from build123d import *

# Parameters (mm, degrees)
F0_R     = 2.5
F0_R_2   = 5
F0_R_3   = 2
F0_W     = 60
F0_H     = 15
F1_DEPTH = 12
F2_R     = 10
F2_R_2   = 9.5
F3_DEPTH = 6
F4_R     = 5
F5_SIZE  = 1


with BuildPart() as f1:
    # F0 (on Top) → F1 (new body)
    with BuildSketch(Plane.XY):
        with BuildLine():
            Line((-165, 140), (-225, 140))
            Line((-225, 140), (-225, -125))
            Line((-225, -125), (-165, -125))
            Line((-165, -125), (-165, -74))
            ThreePointArc((-165, -74), (-168, -71), (-165, -68))
            Line((-165, -68), (-165, -34))
            ThreePointArc((-165, -34), (-168, -31), (-165, -28))
            Line((-165, -28), (-165, 140))
        make_face()
        with Locations((-200, 0)):
            Circle(F0_R, mode=Mode.SUBTRACT)
        with BuildLine():
            Line((165, 140), (-165, 140))
            Line((-165, 140), (-165, -28))
            ThreePointArc((-165, -28), (-162.87868, -28.87868), (-162, -31))
            ThreePointArc((-162, -31), (-162.87868, -33.12132), (-165, -34))
            Line((-165, -34), (-165, -68))
            ThreePointArc((-165, -68), (-162.87868, -68.87868), (-162, -71))
            ThreePointArc((-162, -71), (-162.87868, -73.12132), (-165, -74))
            Line((-165, -74), (-165, -125))
            Line((-165, -125), (-130, -125))
            ThreePointArc((-130, -125), (-125, -120), (-120, -125))
            Line((-120, -125), (120, -125))
            ThreePointArc((120, -125), (125, -120), (130, -125))
            Line((130, -125), (165, -125))
            Line((165, -125), (165, -74))
            ThreePointArc((165, -74), (162, -71), (165, -68))
            Line((165, -68), (165, -34))
            ThreePointArc((165, -34), (162, -31), (165, -28))
            Line((165, -28), (165, 140))
        make_face()
        with BuildLine():
            ThreePointArc((-148, 2), (-146, 0), (-148, -2))
            Line((-148, -2), (-152, -2))
            ThreePointArc((-152, -2), (-154, 0), (-152, 2))
            Line((-152, 2), (-148, 2))
        make_face(mode=Mode.SUBTRACT)
        with Locations((-100, 0)):
            Circle(F0_R, mode=Mode.SUBTRACT)
        with Locations((-125, 125)):
            Circle(F0_R_2, mode=Mode.SUBTRACT)
        Circle(F0_R, mode=Mode.SUBTRACT)
        with Locations((100, 0)):
            Circle(F0_R, mode=Mode.SUBTRACT)
        with Locations((150, 0)):
            Circle(F0_R_3, mode=Mode.SUBTRACT)
        with Locations((125, 125)):
            Circle(F0_R_2, mode=Mode.SUBTRACT)
        with Locations((-195, -132.5)):
            Rectangle(F0_W, F0_H)
        with BuildLine():
            Line((225, 140), (165, 140))
            Line((165, 140), (165, -28))
            ThreePointArc((165, -28), (167.12132, -28.87868), (168, -31))
            ThreePointArc((168, -31), (167.12132, -33.12132), (165, -34))
            Line((165, -34), (165, -68))
            ThreePointArc((165, -68), (167.12132, -68.87868), (168, -71))
            ThreePointArc((168, -71), (167.12132, -73.12132), (165, -74))
            Line((165, -74), (165, -125))
            Line((165, -125), (225, -125))
            Line((225, -125), (225, 140))
        make_face()
        with Locations((200, 0)):
            Circle(F0_R, mode=Mode.SUBTRACT)
        with BuildLine():
            Line((-130, -125), (-165, -125))
            Line((-165, -125), (-165, -140))
            Line((-165, -140), (165, -140))
            Line((165, -140), (165, -125))
            Line((165, -125), (130, -125))
            ThreePointArc((130, -125), (125, -130), (120, -125))
            Line((120, -125), (-120, -125))
            ThreePointArc((-120, -125), (-125, -130), (-130, -125))
        make_face()
        with Locations((195, -132.5)):
            Rectangle(F0_W, F0_H)
    extrude(amount=F1_DEPTH)

    # F2 (on face) → F3 (cut)
    with BuildSketch(Plane(origin=(0, 0, 0), x_dir=(1, 0, 0), z_dir=(0, 0, -1))):
        with Locations((-165, 71)):
            Circle(F2_R)
        with Locations((165, 71)):
            Circle(F2_R)
        with Locations((165, 31)):
            Circle(F2_R)
        with Locations((-165, 31)):
            Circle(F2_R)
        with Locations((-100, 0)):
            Circle(F2_R_2)
        with Locations((-200, 0)):
            Circle(F2_R_2)
        with Locations((100, 0)):
            Circle(F2_R_2)
        Circle(F2_R_2)
        with Locations((200, 0)):
            Circle(F2_R_2)
    extrude(amount=-F3_DEPTH, mode=Mode.SUBTRACT)

    # F4
    f4_edges = [f1.edges().sort_by_distance(p)[0] for p in [
        (-225, -140, 6),
        (225, -140, 6),
        (225, 140, 6),
        (-225, 140, 6),
    ]]
    fillet(f4_edges, radius=F4_R)

    # F5
    f5_edges = [f1.edges().sort_by_distance(p)[0] for p in [
        (197.5, 0, 6),
        (97.5, 0, 6),
        (-202.5, 0, 6),
        (-102.5, 0, 6),
        (-2.5, 0, 6),
        (165, -68, 6),
        (165, -28, 6),
        (120, 125, 0),
        (-130, 125, 0),
        (-165, -28, 6),
        (-165, -68, 6),
    ]]
    chamfer(f5_edges, length=F5_SIZE)


solid = f1.part
Geometry: final body of the model. Coordinates: model frame, mm. A direction names the side the tool comes from. Give positions to 0.01 mm unless a question says otherwise; leave off trailing zeros. Write each loop counter-clockwise with the first axis right and the second up, starting at its lowest first coordinate (ties: lowest second). Pieces come first, ordered by that corner, then holes.
(1) Cut plane C-C, the plane z = 3. Give the number of separate pieces and of enclosed holes in the cut face, then the cut area to 3 significant figures.
(2) Cut plane B-B, the plane x = 125. Return loops of the section in (y, z).
(3) Cut plane A-A, the plane y = 125. Return loops of the section in (x, z).
(4) Access query for faces 5 (the cylindrical face through (-190.939, -2.854, 2.958)), 6 (the flat face through (3, 140, 6)). Directions: +Z, -Z, +X, -X, +Y, -Y. A direction counts if a zero-diameter tool reaches every point of the face in a straight line with its end or side. Return the directions, or none.
(5) Mould query, pull axis Y, two halves, no side actions, for faces 1 (the cylindrical face through (209.061, -2.854, 2.958)), 2 (the flat face through (225, -2, 6)), 3 (the flat face through (4, 0, 6)), 4 (the flat face through (-3, -140, 6)). Classes: released by +Y, released by -Y, zero draft, split by the parting line, or undercut.
(6) First-contact query: P1, Ø6, axis at x = -125, y = 125, coming from the -Z side; P2, Ø6, axis at x = 100, y = 0, coming from the -Z side. Flat tips, straight axial feed; report the tip coordinate or a pass-through.
(7) Ray query, line 1 (Y direction, x = 125, z = 5); line 2 (Y direction, x = -165, z = 4.7); line 3 (X direction, y = 125.5, z = 11). Return the intervals inside material, ascending.
Values follow:
1. separate pieces: 1
1. enclosed holes: 15
1. area: 123,000 mm2
2. outline: (-140, 0) - (-130, 0) - (-130, 12) - (-140, 12) - close; (-120, 0) - (119, 0) - (120, 1) - (120, 12) - (-120, 12) - close; (130, 1) - (131, 0) - (140, 0) - (140, 12) - (130, 12) - close
3. outline: (-225, 0) - (-131, 0) - (-130, 1) - (-130, 12) - (-225, 12) - close; (-120, 1) - (-119, 0) - (119, 0) - (120, 1) - (120, 12) - (-120, 12) - close; (130, 1) - (131, 0) - (225, 0) - (225, 12) - (130, 12) - close
4. face 5: -Z
4. face 6: +Z, -Z, +X, -X, +Y
5. face 1: undercut
5. face 2: zero draft
5. face 3: undercut
5. face 4: released by -Y
6. P1: passes through
6. P2: stops at z = 6.5
7. line 1: y = -140 to -130, -120 to 120, 130 to 140
7. line 2: y = -140 to -81, -61 to -41, -21 to 140
7. line 3: x = -225 to -129.97, -120.03 to 120.03, 129.97 to 225
